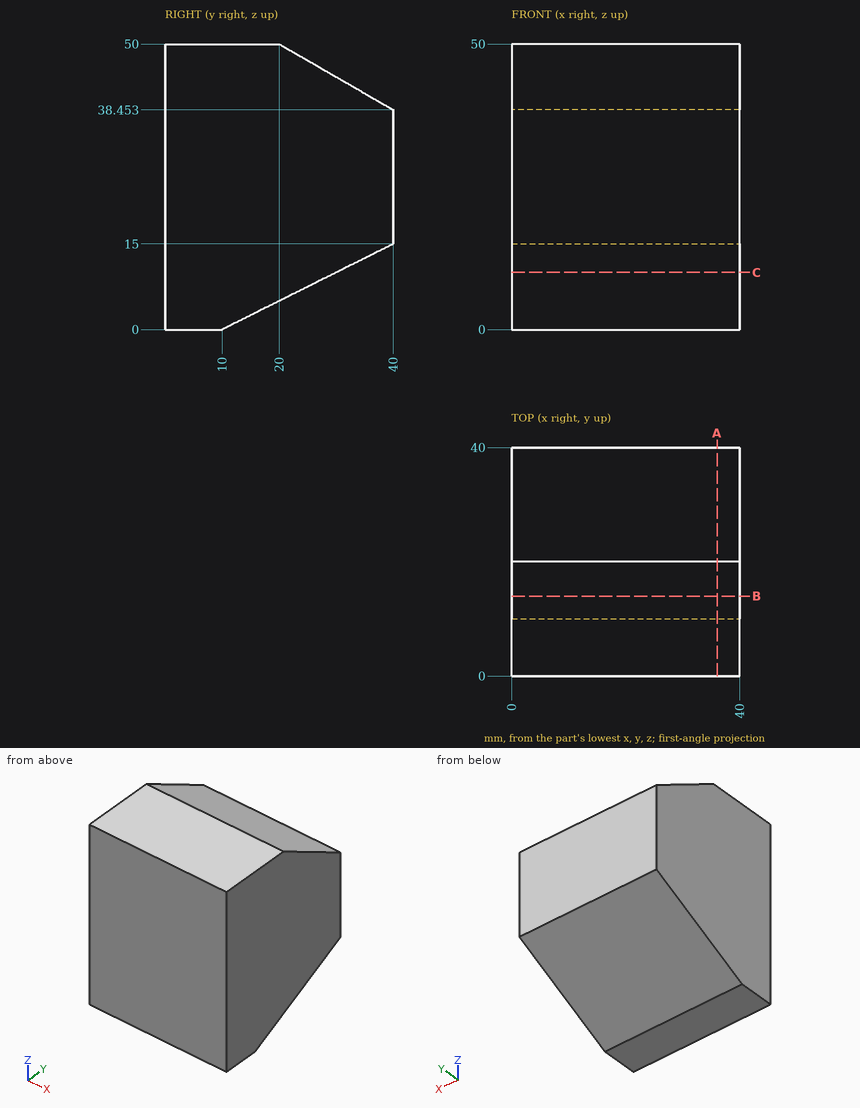
Design review of the part shown in the three views and the two pictorial views. Dimensions are in mm from the part's minimum x, y and z. Coordinates: 2 decimals unless noted, no trailing zeros. Order: outer loops, then holes, each group sorted by start corner. A loop starts at its lowest first (then second) coordinate and runs counter-clockwise, first axis right, second up.
1) Take a section at B-B, the plane y = 14. Give the boundary of the cut face in (x, z), and give its area (3 significant figures).
2) Take a section at C-C, the plane z = 10. Give the boundary of the cut face in (x, y).
3) Wall thickness on line 1 along Z through (x, y) = (30, 35.5); line 2 along Y through (x, z) = (15, 40); line 3 along Y through (x, z) = (15, 13.5): over which ranges is each line inside the solid? List them lowest first.
4) Take a section at A-A, the plane x = 36. Give the boundary of the cut face in (y, z), and give its area (3 significant figures).
5) Clearance check with a flat-ended pin moving along its axis: pin 1 (2 mm diameter, centred on x = 9.5, y = 28, fed in from -Z). State where the tip first meets the part, or that it passes through.
Returned:
1. outline: (0, 2) - (40, 2) - (40, 50) - (0, 50) - close
1. area: 1,920 mm2
2. outline: (0, 0) - (40, 0) - (40, 30) - (0, 30) - close
3. line 1: z = 12.75 to 41.05
3. line 2: y = 0 to 37.32
3. line 3: y = 0 to 37
4. outline: (0, 0) - (10, 0) - (40, 15) - (40, 38.45) - (20, 50) - (0, 50) - close
4. area: 1,660 mm2
5. pin 1: stops at z = 8.5
